```python
from build123d import *

# Parameters (mm, degrees)
SKETCH_1_W                   = 40
SKETCH_1_H                   = 39
EXTRUDE_1_DEPTH              = 20
SKETCH_2_W                   = 20
SKETCH_2_H                   = 2
EXTRUDE_2_DEPTH              = 15
SKETCH_6_W                   = 20
SKETCH_6_H                   = 2
EXTRUDE_3_DEPTH              = 15
SKETCH_8_R                   = 2
CUT_EXTRUDE_1_DEPTH          = 6
SKETCH_11_R                  = 3
EXTRUDE_5_DEPTH              = 1
SKETCH_16_R                  = 1.5
EXTRUDE_7_DEPTH              = 5
HOLE_WIZARD_M3_3_D           = 2.5
HOLE_WIZARD_M3_3_DEPTH       = 3
HOLE_WIZARD_M3_3_CSINK_D     = 2.55
HOLE_WIZARD_M3_3_CSINK_ANGLE = 90
HOLE_WIZARD_M3_3_TIP         = 0.751075774
FILLET_4_R                   = 1


with BuildPart() as part:
    # 草图1 → 凸台-拉伸1 (new body)
    with BuildSketch(Plane.XY):
        Rectangle(SKETCH_1_W, SKETCH_1_H)
    extrude(amount=EXTRUDE_1_DEPTH)

    # 草图2 → 凸台-拉伸2 (add)
    with BuildSketch(Plane.ZY.offset(20)):
        with Locations((10, 10.5)):
            Rectangle(SKETCH_2_W, SKETCH_2_H)
    extrude(amount=EXTRUDE_2_DEPTH)

    # 草图6 → 凸台-拉伸3 (add)
    with BuildSketch(Plane(origin=(20, 0, 0), x_dir=(0, 0, -1), z_dir=(1, 0, 0))):
        with Locations((-10, 10.5)):
            Rectangle(SKETCH_6_W, SKETCH_6_H)
    extrude(amount=EXTRUDE_3_DEPTH)

    # 草图8 → 切除-拉伸1 (cut)
    with BuildSketch(Plane(origin=(0, 11.5, 0), x_dir=(1, 0, 0), z_dir=(0, 1, 0))):
        with Locations(Location((-23.804244171, -5, 0), (0, 0, 270))):
            Circle(SKETCH_8_R)
        with Locations(Location((-23.804244171, -15, 0), (0, 0, 270))):
            Circle(SKETCH_8_R)
        with Locations(Location((24.195755829, -5, 0), (0, 0, 270))):
            Circle(SKETCH_8_R)
        with Locations(Location((24.195755829, -15, 0), (0, 0, 180))):
            Circle(SKETCH_8_R)
    extrude(amount=-CUT_EXTRUDE_1_DEPTH, mode=Mode.SUBTRACT)

    # 草图11 → 凸台-拉伸5 (add)
    with BuildSketch(Plane(origin=(0, 19.5, 0), x_dir=(1, 0, 0), z_dir=(0, 1, 0))):
        with Locations(Location((-9.804244171, -10, 0), (0, 0, 90))):
            Circle(SKETCH_11_R)
    extrude(amount=EXTRUDE_5_DEPTH)

    # 草图16 → 凸台-拉伸7 (add)
    with BuildSketch(Plane(origin=(0, 20.5, 0), x_dir=(1, 0, 0), z_dir=(0, 1, 0))):
        with Locations(Location((-9.804244171, -10, 0), (0, 0, 270))):
            Circle(SKETCH_16_R)
    extrude(amount=EXTRUDE_7_DEPTH)

    # M3 螺纹孔的螺纹孔钻头3
    with Locations(Plane(origin=(0, 25.5, 0), x_dir=(1, 0, 0), z_dir=(0, 1, 0))):
        with Locations((-9.804244171, -10)):
            CounterSinkHole(HOLE_WIZARD_M3_3_D / 2, HOLE_WIZARD_M3_3_CSINK_D / 2, depth=HOLE_WIZARD_M3_3_DEPTH, counter_sink_angle=HOLE_WIZARD_M3_3_CSINK_ANGLE)
            with Locations((0, 0, -(HOLE_WIZARD_M3_3_DEPTH + HOLE_WIZARD_M3_3_TIP / 2))):  # 118° drill point
                Cone(0, HOLE_WIZARD_M3_3_D / 2, HOLE_WIZARD_M3_3_TIP, mode=Mode.SUBTRACT)

    # 圆角4
    fillet_4_edges = [part.edges().sort_by_distance(p)[0] for p in [
        (0, 19.5, 0),
        (-9.804244171, 19.5, 13),
        (-20, 19.5, 10),
        (20, 19.5, 10),
        (0, 19.5, 20),
    ]]
    fillet(fillet_4_edges, radius=FILLET_4_R - 0.0001)  # a hair under: the kernel refuses the full size


solid = part.part
```
Read the model definition and answer for the solid it produces. Units are mm, in the model's axes. A direction names the side the tool comes from. Give positions to 0.01 mm unless a question says otherwise; leave off trailing zeros. Order: outer loops, then holes, each group sorted by start corner. A loop starts at its lowest first (then second) coordinate and runs counter-clockwise, first axis right, second up. Notation, with made-up numbers: (-30.75, 62.25) -> (28.25, 62.25) arc R26 ccw to (28.25, 96.25) -> close; hole circle Ø8 at (25.25, 35.25). An arc over 180 degrees is marked (long way). Write item = value, one per line.
1. Given pin 1 (7.5 mm diameter, centred on x = -31, z = 13.5, fed in from +Y); pin 2 (4 mm diameter, centred on y = -8, z = 13.5, fed in from +X); pin 3 (3.5 mm diameter, centred on x = -23.8, z = 15, fed in from -Y); pin 4 (4.5 mm diameter, centred on x = -26, z = 13, fed in from -Y), each flat-ended and moving along its own axis, determine where each tip first touches the part or whether it passes through.
Numbers:
pin_1 = 11.5
pin_2 = 20
pin_3 = through
pin_4 = 9.5
2. A cutting plane is placed at A-A, the plane z = 5. Write down the section's boundary in (x, y).
Numbers:
outline = (-35, 9.5) -> (-25.8, 9.5) -> (-25.8, 11.5) -> (-35, 11.5) -> close; (-21.8, 9.5) -> (-20, 9.5) -> (-20, -19.5) -> (20, -19.5) -> (20, 9.5) -> (22.2, 9.5) -> (22.2, 11.5) -> (20, 11.5) -> (20, 18.5) arc R1 ccw to (19, 19.5) -> (-19, 19.5) arc R1 ccw to (-20, 18.5) -> (-20, 11.5) -> (-21.8, 11.5) -> close; (26.2, 9.5) -> (35, 9.5) -> (35, 11.5) -> (26.2, 11.5) -> close
3. A cutting plane is placed at C-C, the plane z = 16.25. Write down the section's boundary in (x, y), and give its area (3 significant figures).
Numbers:
outline = (-35, 9.5) -> (-25.37, 9.5) -> (-25.37, 11.5) -> (-35, 11.5) -> close; (-22.24, 9.5) -> (-20, 9.5) -> (-20, -19.5) -> (20, -19.5) -> (20, 9.5) -> (22.63, 9.5) -> (22.63, 11.5) -> (20, 11.5) -> (20, 18.5) arc R1 ccw to (19, 19.5) -> (-19, 19.5) arc R1 ccw to (-20, 18.5) -> (-20, 11.5) -> (-22.24, 11.5) -> close; (25.76, 9.5) -> (35, 9.5) -> (35, 11.5) -> (25.76, 11.5) -> close
area = 1,610 mm²
4. The mould has two halves that part along X. Classify faces 5 (the face through (-20, 15, 10)), 6 (the face through (27, 11.5, 10)), 7 (the face through (35, 11, 10)), 8 (the face through (-21.82, 10.51, 14.74)): +X half, -X half, draft (parallel to the pull), parting line (faces both ways), or undercut.
Numbers:
face_5 = -X half
face_6 = draft
face_7 = +X half
face_8 = undercut
5. A cutting plane is placed at D-D, the plane y = 7. Write down the section's boundary in (x, z), and give its area (3 significant figures).
Numbers:
outline = (-20, 0) -> (20, 0) -> (20, 20) -> (-20, 20) -> close
area = 800 mm²
6. Straight lines are drawn through the part: line 1 along X through (y, z) = (10.15, 5); line 2 along X through (y, z) = (-6, 3); line 3 along X through (y, z) = (23.25, 10). For each, find the intervals that lie inside material, in ascending order.
Numbers:
line_1 = -35 to -25.8, -21.8 to 22.2, 26.2 to 35
line_2 = -20 to 20
line_3 = -11.3 to -11.05, -8.55 to -8.3
7. For faces 1 (the face through (27, 9.5, 10)), 2 (the face through (-35, 11, 10)), 3 (the face through (-20, -5, 10)), 4 (the face through (-8.5, 20.5, 8.7)), determine the directions among +Z, -Z, +X, -X, +Y, -Y from which every point of the face is accessible in a straight line to the end or side of a thin tool.
Numbers:
face_1 = +Z, -Z, +X, -Y
face_2 = +Z, -Z, -X, +Y, -Y
face_3 = +Z, -Z, -X, -Y
face_4 = +Y
8. A cutting plane is placed at B-B, the plane x = 10.5. Write down the section's boundary in (y, z).
Numbers:
outline = (-19.5, 0) -> (18.5, 0) arc R1 ccw to (19.5, 1) -> (19.5, 19) arc R1 ccw to (18.5, 20) -> (-19.5, 20) -> close
